The model under review builds one solid part; all positions refer to its coordinate system, in mm. A direction names the side the tool comes from. Coordinates: 2 decimals unless noted, no trailing zeros. Order: outer loops, then holes, each group sorted by start corner. A loop starts at its lowest first (then second) coordinate and runs counter-clockwise, first axis right, second up. Notation, with made-up numbers: M 50,70 L 58,70 A25 cw 58,84 Z; hole C 81,68 d5. An arc over 180 degrees is marked long. Answer in a Markdown table with one row per item.
from build123d import *

# Parameters (mm, degrees)
BOSS_EXTRUDE1_DEPTH       = 20
SKETCH4_W                 = 17.215870058
SKETCH4_H                 = 6
BOSS_EXTRUDE2_DEPTH       = 1
BOSS_EXTRUDE3_DEPTH       = 3.6
F_1_0MM_DOWEL_HOLE1_D     = 0.5
F_1_0MM_DOWEL_HOLE1_DEPTH = 4.6


with BuildPart() as part:
    # Sketch3 → Boss-Extrude1 (new body)
    with BuildSketch(Plane(origin=(-3.4e-08, 0.000254638, -31.967040172), x_dir=(1, 0, -1e-09), z_dir=(1e-09, -7.966e-06, 1))):
        Polygon((98.980598041, 85.65676806), (114.480598041, 85.65676806), (114.480601842, 91.65676711), (112.980601807, 91.65676806), (112.980601807, 86.65676806), (100.480601842, 86.65676806), (100.480601842, 91.65676806), (98.980601842, 91.65676806), align=None)
    extrude(amount=BOSS_EXTRUDE1_DEPTH)

    # Sketch4 → Boss-Extrude2 (add)
    with BuildSketch(Plane(origin=(-1.3e-08, 9.5325e-05, -11.967040173), x_dir=(1, 0, -1e-09), z_dir=(1e-09, -7.966e-06, 1))):
        with Locations((106.672666813, 88.65676806)):
            Rectangle(SKETCH4_W, SKETCH4_H)
    extrude(amount=BOSS_EXTRUDE2_DEPTH)

    # Sketch7 → Boss-Extrude3 (add)
    with BuildSketch(Plane(origin=(-1.3e-08, 9.5325e-05, -11.967040173), x_dir=(-1, 0, 1e-09), z_dir=(-1e-09, 7.966e-06, -1))):
        Polygon((-112.980601816, 91.65676806), (-112.980601825, 86.65676806), (-100.480601842, 86.65676806), (-100.480601851, 91.65676806), align=None)
    extrude(amount=BOSS_EXTRUDE3_DEPTH)

    # Ø1.0mm Dowel Hole1
    with Locations(Plane(origin=(-1.2e-08, 8.7359e-05, -10.967040173), x_dir=(1, 0, -1e-09), z_dir=(1e-09, -7.966e-06, 1))):
        with Locations((106.672666813, 90.15676806)):
            Hole(F_1_0MM_DOWEL_HOLE1_D / 2, depth=F_1_0MM_DOWEL_HOLE1_DEPTH)


solid = part.part
(1) To check wall thickness, follow line 1 (X direction, y = 91, z = -28.25); line 2 (Z direction, x = 112, y = 87.5); line 3 (Y direction, x = 102.5, z = -26.25). State the ranges of each line that lie inside material, in increasing order. Write a range as [from, to].
Report:
| item | result |
|---|---|
| line 1 | [98.98, 100.48], [112.98, 114.48] |
| line 2 | [-15.57, -10.97] |
| line 3 | [85.66, 86.66] |
(2) Machinability: for faces 4 (the flat face through (98.065, 88.6, -11.5)), 5 (the flat face through (100.481, 89, -24)), which of the approach directions +Z, -Z, +X, -X, +Y, -Y give a long, thin tool a straight path to every point of the face, cutting with its end or side? Answer none if there is none.
Report:
| item | result |
|---|---|
| face 4 | +Z, -Z, -X, +Y, -Y |
| face 5 | -Z, +Y |
(3) The part is to be moulded in two halves that separate along X. For faces 1 (the flat face through (112.981, 89, -24)), 2 (the flat face through (114.481, 89, -22)), 3 (the flat face through (98.981, 89, -22)), say which applies: +X half, -X half, draft (parallel to the pull), parting line (faces both ways), or undercut.
Report:
| item | result |
|---|---|
| face 1 | undercut |
| face 2 | +X half |
| face 3 | -X half |
(4) Take a section at C-C (z = -24.5). Write out the cut boundary in (x, y).
Report:
| item | result |
|---|---|
| outline | M 98.98,85.66 L 114.48,85.66 L 114.48,91.66 L 112.98,91.66 L 112.98,86.66 L 100.48,86.66 L 100.48,91.66 L 98.98,91.66 Z |
(5) Take a section at B-B (y = 91). Write out the cut boundary in (x, z), then the cut area to 3 significant figures.
Report:
| item | result |
|---|---|
| outline | M 98.06,-11.97 L 98.98,-11.97 L 98.98,-31.97 L 100.48,-31.97 L 100.48,-15.57 L 112.98,-15.57 L 112.98,-31.97 L 114.48,-31.97 L 114.48,-11.97 L 115.28,-11.97 L 115.28,-10.97 L 98.06,-10.97 Z |
| area | 122 mm^2 |
(6) Insertion check: P1, Ø3, axis at y = 89, z = -21, coming from the -X side; P2, Ø2, axis at x = 111, z = -27, coming from the +Y side; P3, Ø3, axis at y = 91, z = -18.5, coming from the +X side. Each pin has a flat end and moves straight along its axis. Give the tip position at first contact, or say it passes through.
Report:
| item | result |
|---|---|
| P1 | x = 98.98 |
| P2 | y = 86.66 |
| P3 | x = 114.48 |
(7) Take a section at A-A (x = 107.5). Write out the cut boundary in (y, z), then the cut area to 3 significant figures.
Report:
| item | result |
|---|---|
| outline | M 85.66,-31.97 L 86.66,-31.97 L 86.66,-15.57 L 91.66,-15.57 L 91.66,-10.97 L 85.66,-10.97 Z |
| area | 44.0 mm^2 |
